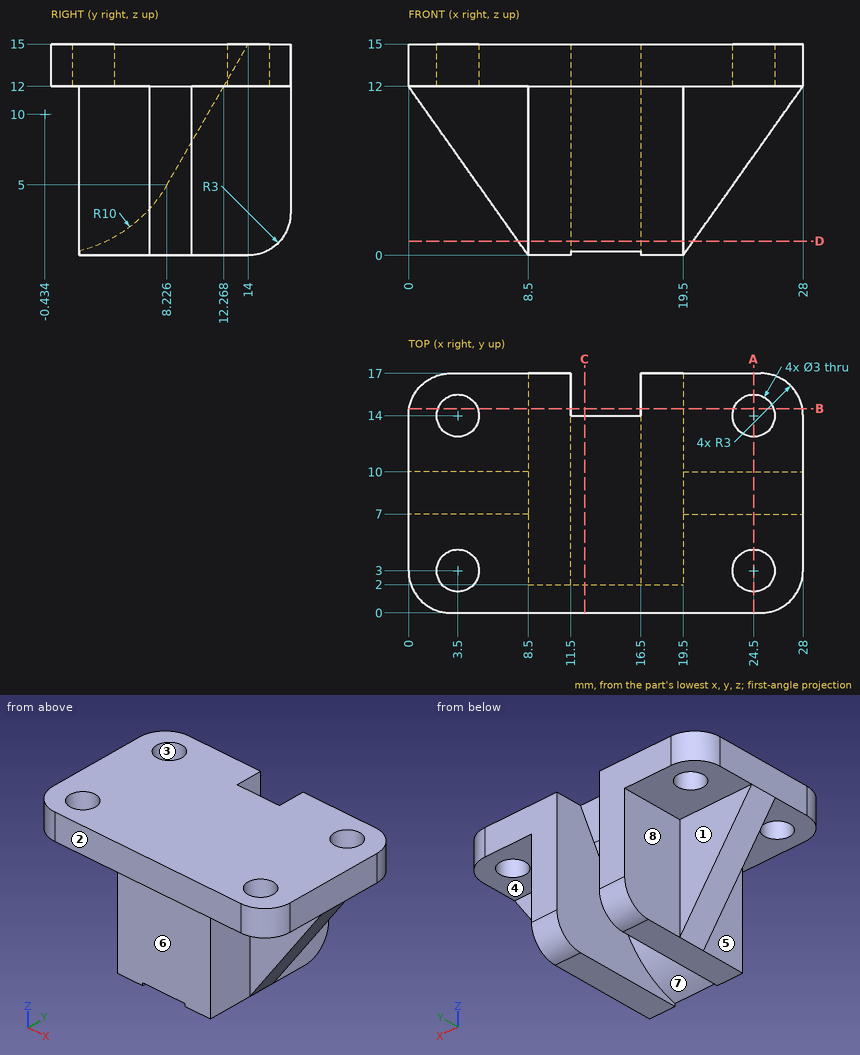
Study the drawing (mm; zero at the part's minimum x, y, z) and answer. A direction names the side the tool comes from. Give positions to 0.01 mm unless a question says otherwise; leave off trailing zeros. Write each loop counter-clockwise with the first axis right and the second up, starting at its lowest first coordinate (ties: lowest second). Pieces come first, ordered by that corner, then holes. Notation, with made-up numbers: (-23, 18.5) - (23, 18.5) arc R28 cw to (23, 54.5) - close; hole circle Ø9 at (80, -3.5). An arc over 180 degrees is marked (long way). Write item = value, one per line. Start each with the question number.
Item 1: Find section C-C (x = 12.5). Give the vertices of the cut face in (y, z).
Item 2: A tool of negligible diameter and unlimited length cuts with its end or side. For the marked faces 4, 5, 6, 7 and 8, from which of +Z, -Z, +X, -X, +Y, -Y can it reach the whole face along a straight path? Write none if from no direction.
Item 3: Find section B-B (y = 14.5). Give the vertices of the cut face in (x, z) (1 decimal).
Item 4: Find the intervals of material crossed by probe 1 along Y at (x, z) = (24.5, 14.35); probe 2 along X at (y, z) = (12, 1.25); probe 3 along X at (y, z) = (14.5, 14.25) (1 decimal), in increasing order. Write a range as [from, to].
Item 5: The mould has two halves that part along Y. Classify the marked faces 1, 2 and 3: +Y half, -Y half, draft (parallel to the pull), parting line (faces both ways), or undercut.
Item 6: Find section A-A (x = 24.5). Give the vertices of the cut face in (y, z).
Item 7: Find section D-D (z = 1). Give the vertices of the cut face in (x, y) (1 decimal).
Item 8: Each of these flat-tipped pins is pushed along its axis until it touches: P1, Ø4, axis at x = 4.5, z = 5, coming from the -Y side; P2, Ø7.5, axis at y = 11.5, z = 11, coming from the -X side; P3, Ø3.5, axis at x = 4, y = 12.5, coming from the -Z side; P4, Ø7, axis at x = 24, z = 5.5, coming from the +Y side. Where does it stop, or does it pass through?
Response:
q1.outline = (0, 12) - (2, 12) - (2, 0.3) arc R10 ccw to (8.23, 5) - (14, 15) - (0, 15) - close
q2.face_4 = -Z, +X, +Y
q2.face_5 = -Z, -X, -Y
q2.face_6 = -Z, +X, -X, -Y
q2.face_7 = -Z, +Y
q2.face_8 = -Z, -X, +Y
q3.outline = (0, 12) - (2.1, 12) - (2.1, 15) - (0, 15) - close; (4.9, 12) - (8.5, 12) - (8.5, 0) - (11.5, 0) - (11.5, 15) - (4.9, 15) - close; (16.5, 0) - (19.5, 0) - (19.5, 12) - (23.1, 12) - (23.1, 15) - (16.5, 15) - close; (25.9, 12) - (28, 12) - (28, 15) - (25.9, 15) - close
q4.probe_1 = [0, 1.5], [4.5, 12.5], [15.5, 17]
q4.probe_2 = [8.5, 11.5], [16.5, 19.5]
q4.probe_3 = [0, 2.1], [4.9, 11.5], [16.5, 23.1], [25.9, 28]
q5.face_1 = +Y half
q5.face_2 = -Y half
q5.face_3 = undercut
q6.outline = (0, 12) - (1.5, 12) - (1.5, 15) - (0, 15) - close; (4.5, 12) - (7, 12) - (7, 7.06) - (10, 7.06) - (10, 12) - (12.5, 12) - (12.5, 15) - (4.5, 15) - close; (15.5, 12) - (17, 12) - (17, 15) - (15.5, 15) - close
q7.outline = (7.8, 7) - (8.5, 7) - (8.5, 2) - (19.5, 2) - (19.5, 7) - (20.2, 7) - (20.2, 10) - (19.5, 10) - (19.5, 16.2) - (16.5, 16.2) - (16.5, 3.9) - (11.5, 3.9) - (11.5, 16.2) - (8.5, 16.2) - (8.5, 10) - (7.8, 10) - close
q8.P1 = 7
q8.P2 = 0
q8.P3 = 12
q8.P4 = 10
